For this review, use the dimensioned drawing (mm, ordinates from the lowest corner) and the shaded views. Give positions to 0.01 mm unless a question says otherwise; leave off trailing zeros. Loops run counter-clockwise (first coordinate to the right, second up) from the corner with the lowest first, then second, coordinate; pieces in that order, holes last. Notation, with made-up numbers: M -26.75,83.25 L 28.25,83.25 A15 cw 28.25,97.25 Z; hole C 58,-35 d7. An arc over 180 degrees is marked long. Use CSV: the item, a comma, the result in double quotes. Start each with the question number.
1. Take a section at C-C, the plane z = 3.7. State how many separate pieces and enclosed holes the cut face has, and give its area (3 significant figures).
2. Take a section at D-D, the plane x = 28.5. Write out the cut boundary in (y, z).
3. Take a section at B-B, the plane x = 5. Write out the cut boundary in (y, z), and give its area (3 significant figures).
4. The part is to be moulded in two halves that separate along Y. For the marked faces 1, 2 and 3, say which applies: pulls with the +Y half, pulls with the -Y half, needs draft (parallel to the pull), parting line crosses it, or undercut.
5. Take a section at A-A, the plane y = 35.8. Write out the cut boundary in (x, z).
6. To check wall thickness, follow line 1 (Y direction, x = 29.5, z = 1.35); line 2 (Y direction, x = 29, z = 1.9) (1 decimal); line 3 (X direction, y = 14.5, z = 1.05) (1 decimal). State the ranges of each line that lie inside material, in increasing order. Write a range as [from, to].
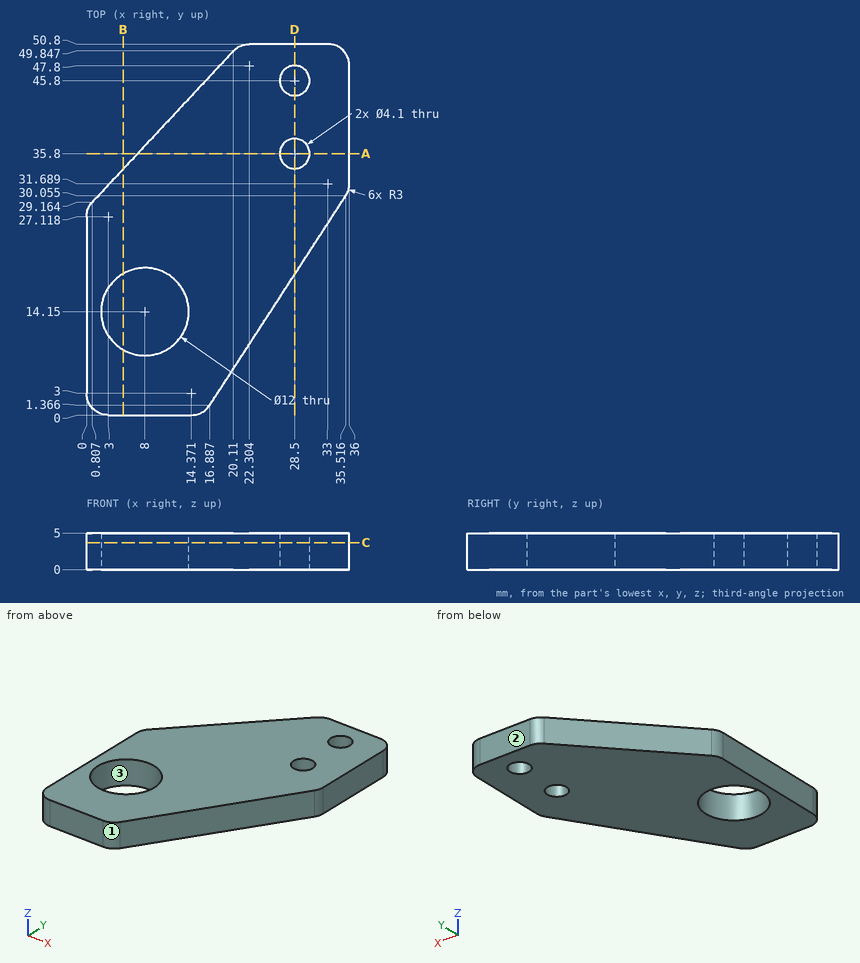
Result set:
1,separate pieces,"1"
1,enclosed holes,"3"
1,area,"1,140 mm2"
2,outline,"M 19.25,0 L 33.75,0 L 33.75,5 L 19.25,5 Z; M 37.85,0 L 43.75,0 L 43.75,5 L 37.85,5 Z; M 47.85,0 L 50.8,0 L 50.8,5 L 47.85,5 Z"
3,outline,"M 0,0 L 8.95,0 L 8.95,5 L 0,5 Z; M 19.35,0 L 33.66,0 L 33.66,5 L 19.35,5 Z"
3,area,"116 mm2"
4,face 1,"pulls with the -Y half"
4,face 2,"pulls with the +Y half"
4,face 3,"undercut"
5,outline,"M 7,0 L 26.45,0 L 26.45,5 L 7,5 Z; M 30.55,0 L 36,0 L 36,5 L 30.55,5 Z"
6,line 1,"[20.79, 34.01], [37.59, 44.01], [47.59, 50.8]"
6,line 2,"[20, 33.8], [37.8, 43.8], [47.8, 50.8]"
6,line 3,"[0, 2], [14, 25.4]"
